The model under review builds one solid part; all positions refer to its coordinate system, in mm. Face numbers are marked on the shaded views. A direction names the side the tool comes from. Give positions to 0.01 mm unless a question says otherwise; leave off trailing zeros. Loops run counter-clockwise (first coordinate to the right, second up) from the corner with the lowest first, then second, coordinate; pieces in that order, holes last. Notation, with made-up numbers: M 53,64 L 108,64 A18 cw 108,88 Z; hole C 79,62.5 d4. An arc over 180 degrees is marked long. Return JSON: item names as keys, results as strings.
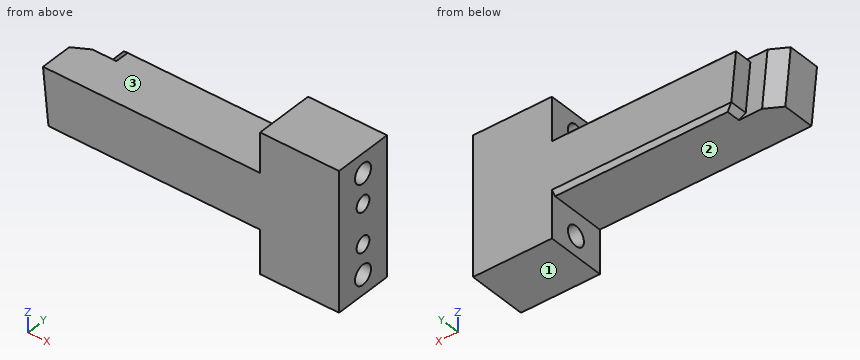
```python
from build123d import *

# Parameters (mm, degrees)
F0_W     = 6
F0_H     = 4
F0_W_2   = 20
F0_H_2   = 5
F1_DEPTH = 10.5
F2_W     = 20
F2_H     = 5
F3_DEPTH = 4.5
F4_R     = 2.5
F5_DEPTH = 20.001
F6_R     = 2
F7_DEPTH = 6
F8_SIZE  = 1
F9_SIZE2 = 2.3094010768
F9_SIZE  = 4


with BuildPart() as f1:
    # F0 (on Front) → F1 (new body)
    with BuildSketch(Plane.XZ):
        Polygon((66.887199, -59.346183), (72.887199, -59.346183), (72.887199, -55.346183), (66.887199, -55.346183), (66.887199, -57.346183), align=None)
        Polygon((52.887199, -45.846183), (6.252832, -45.846183), (7.441181, -57.846183), (52.887199, -57.846183), (52.887199, -58.846183), (52.887199, -64.846183), (72.887199, -64.846183), (72.887199, -59.346183), (66.887199, -59.346183), (65.732498, -57.346183), (66.887199, -55.346183), (72.887199, -55.346183), (72.887199, -49.346183), (66.887199, -49.346183), (65.732498, -47.346183), (66.887199, -45.346183), (72.887199, -45.346183), (72.887199, -39.846183), (52.887199, -39.846183), (52.887199, -44.846183), align=None)
        with Locations((69.887199, -47.346183)):
            Rectangle(F0_W, F0_H)
        with Locations((62.887199, -37.346183)):
            Rectangle(F0_W_2, F0_H_2)
        with Locations((62.887199, -67.346183)):
            Rectangle(F0_W_2, F0_H_2)
        Polygon((2.754653, -58.846183), (1.368245, -44.846183), (-2.112801, -44.846183), (-0.726393, -58.846183), align=None)
        Polygon((7.984883, -44.846183), (1.368245, -44.846183), (2.754653, -58.846183), (9.173232, -58.846183), (7.441181, -57.846183), (6.252832, -45.846183), align=None)
        Polygon((52.887199, -44.846183), (7.984883, -44.846183), (6.252832, -45.846183), (52.887199, -45.846183), align=None)
        Polygon((7.441181, -57.846183), (9.173232, -58.846183), (52.887199, -58.846183), (52.887199, -57.846183), align=None)
        Polygon((65.732498, -57.346183), (66.887199, -59.346183), (66.887199, -57.346183), align=None)
        Polygon((66.887199, -49.346183), (66.887199, -45.346183), (65.732498, -47.346183), align=None)
        Polygon((65.732498, -57.346183), (66.887199, -57.346183), (66.887199, -55.346183), align=None)
    extrude(amount=-F1_DEPTH)

    # F2 (on face) → F3 (join)
    with BuildSketch(Plane(origin=(0, 10.5, 0), x_dir=(-1, 0, 0), z_dir=(0, 1, 0))):
        with Locations((-62.887199, -37.346183)):
            Rectangle(F2_W, F2_H)
        Polygon((-72.887199, -55.346183), (-72.887199, -59.346183), (-72.887199, -64.846183), (-52.887199, -64.846183), (-52.887199, -58.846183), (-9.173232, -58.846183), (-7.441181, -57.846183), (-6.252832, -45.846183), (-7.984883, -44.846183), (-52.887199, -44.846183), (-52.887199, -39.846183), (-72.887199, -39.846183), (-72.887199, -45.346183), (-72.887199, -49.346183), align=None)
        with Locations((-62.887199, -67.346183)):
            Rectangle(F2_W, F2_H)
    extrude(amount=F3_DEPTH)

    # F4 (on face) → F5 (cut, through all)
    with BuildSketch(Plane(origin=(52.887199, 0, 0), x_dir=(0, -1, 0), z_dir=(-1, 0, 0))):
        with Locations((-7.5, -39.846183)):
            Circle(F4_R)
        with Locations((-7.5, -64.846183)):
            Circle(F4_R)
    extrude(amount=-F5_DEPTH, mode=Mode.SUBTRACT)

    # F6 (on face) → F7 (cut)
    with BuildSketch(Plane.YZ.offset(72.887199)):
        with Locations((7.5, -47.346183)):
            Circle(F6_R)
        with Locations((7.5, -57.346183)):
            Circle(F6_R)
    extrude(amount=-F7_DEPTH, mode=Mode.SUBTRACT)

    # F8
    f8_edges = [f1.edges().sort_by_distance(p)[0] for p in [
        (30.436041, 15, -44.846183),
        (31.030216, 15, -58.846183),
    ]]
    chamfer(f8_edges, length=F8_SIZE)

    # F9
    f9_edges = [f1.edges().sort_by_distance(p)[0] for p in [
        (-1.419597, 10.5, -51.846183),
    ]]
    f9_side = f1.faces().sort_by_distance((2.782636, 10.5, -51.840563))[0]
    chamfer(f9_edges, length=F9_SIZE, length2=F9_SIZE2, reference=f9_side)


solid = f1.part
```
1) Consider section B-B on x = 24. Write out the cut boundary in (y, z), then the cut area to 3 significant figures.
From the geometry:
{"outline": "M 0,-58.85 L 14,-58.85 L 15,-57.85 L 15,-45.85 L 14,-44.85 L 0,-44.85 Z", "area": "209 mm²"}
2) Consider section A-A on y = 7.5. Write out the cut boundary in (x, z).
From the geometry:
{"outline": "M -2.11,-44.85 L -0.73,-58.85 L 52.89,-58.85 L 52.89,-62.35 L 72.89,-62.35 L 72.89,-59.35 L 66.89,-59.35 L 66.89,-55.35 L 72.89,-55.35 L 72.89,-49.35 L 66.89,-49.35 L 66.89,-45.35 L 72.89,-45.35 L 72.89,-42.35 L 52.89,-42.35 L 52.89,-44.85 Z; M 52.89,-69.85 L 72.89,-69.85 L 72.89,-67.35 L 52.89,-67.35 Z; M 52.89,-37.35 L 72.89,-37.35 L 72.89,-34.85 L 52.89,-34.85 Z"}
3) Consider section C-C on y = 1.5. Write out the cut boundary in (x, z).
From the geometry:
{"outline": "M -2.11,-44.85 L -0.73,-58.85 L 52.89,-58.85 L 52.89,-69.85 L 72.89,-69.85 L 72.89,-34.85 L 52.89,-34.85 L 52.89,-44.85 Z"}
4) Wall thickness on L1, parallel to Z at x = 70.85, y = 7.5; L2, parallel to Z at x = 59, y = 7.5; L3, parallel to Z at x = 30, y = 3.75: over which ranges is each line inside the solid? List them lowest first. Write a range as from..to.
From the geometry:
{"L1": "-69.85..-67.35, -62.35..-59.35, -55.35..-49.35, -45.35..-42.35, -37.35..-34.85", "L2": "-69.85..-67.35, -62.35..-42.35, -37.35..-34.85", "L3": "-58.85..-44.85"}
5) Insertion check: pin 1 (3.5 mm diameter, centred on y = 7.5, z = -57.35, fed in from -X); pin 2 (4 mm diameter, centred on x = 13.5, y = 9, fed in from +Z); pin 3 (2 mm diameter, centred on x = 4, z = -53, fed in from +Y); pin 4 (4.5 mm diameter, centred on y = 7.5, z = -39.85, fed in from -X). Each pin has a flat end and moves straight along its axis. Give the tip position at first contact, or say it passes through.
From the geometry:
{"pin 1": "x = -1.05", "pin 2": "z = -44.85", "pin 3": "y = 10.5", "pin 4": "through"}
6) Tool access review of the marked faces 1, 2 and 3: name each direction out of +Z, -Z, +X, -X, +Y, -Y from which nothing blocks a thin tool from reaching the whole face with its end or side.
From the geometry:
{"face 1": "-Z, +X, -X, +Y, -Y", "face 2": "-Z, -X, +Y, -Y", "face 3": "+Z, -X, +Y, -Y"}
7) Consider section D-D on x = 64. Write out the cut boundary in (y, z), then the cut area to 3 significant figures.
From the geometry:
{"outline": "M 0,-69.85 L 15,-69.85 L 15,-34.85 L 0,-34.85 Z; hole C 7.5,-64.85 d5; hole C 7.5,-39.85 d5", "area": "486 mm²"}
